from build123d import *

# Parameters (mm, degrees)
SKETCH1_R           = 1.5
BOSS_EXTRUDE1_DEPTH = 27.5
SKETCH1_3_R         = 3.5
BOSS_EXTRUDE2_DEPTH = 18
FILLET1_R           = 0.3
CUT_EXTRUDE1_START  = 6
SKETCH2_W           = 18
SKETCH2_H           = 4.33028374
CUT_EXTRUDE1_DEPTH  = 48


with BuildPart() as part:
    # Sketch1 → Boss-Extrude1 (new body)
    with BuildSketch(Plane(origin=(0, 0, 0), x_dir=(0, 0, -1), z_dir=(1, 0, 0))):
        with BuildLine():
            Line((-0.4375, 4.980822598), (-40.13125, 1.494246779))
            ThreePointArc((-40.13125, 1.494246779), (-38.986805794, 1.10609109), (-38.5, 0))
            ThreePointArc((-38.5, 0), (-38.986805794, -1.10609109), (-40.13125, -1.494246779))
            Line((-40.13125, -1.494246779), (-0.4375, -4.980822598))
            ThreePointArc((-0.4375, -4.980822598), (-5, 0), (-0.4375, 4.980822598))
        make_face()
        with Locations((-40, 0)):
            Circle(SKETCH1_R)
    extrude(amount=BOSS_EXTRUDE1_DEPTH)

    # Sketch1_3 → Boss-Extrude2 (add)
    with BuildSketch(Plane(origin=(0, 0, 0), x_dir=(0, 0, -1), z_dir=(1, 0, 0))):
        with BuildLine():
            Line((-0.4375, 4.980822598), (-40.13125, 1.494246779))
            ThreePointArc((-40.13125, 1.494246779), (-41.5, 0), (-40.13125, -1.494246779))
            Line((-40.13125, -1.494246779), (-0.4375, -4.980822598))
            ThreePointArc((-0.4375, -4.980822598), (5, 0), (-0.4375, 4.980822598))
        make_face()
        Circle(SKETCH1_3_R, mode=Mode.SUBTRACT)
    extrude(amount=-BOSS_EXTRUDE2_DEPTH)

    # Fillet1
    fillet1_edges = [part.edges().sort_by_distance(p)[0] for p in [
        (13.75, 4.980822598, 0.4375),
        (13.75, -4.980822598, 0.4375),
    ]]
    fillet(fillet1_edges, radius=FILLET1_R)

    # Sketch2 → Cut-Extrude1 (cut)
    with BuildSketch(Plane.XY.offset(CUT_EXTRUDE1_START)):
        with Locations((-9, -3.96514187)):
            Rectangle(SKETCH2_W, SKETCH2_H)
    extrude(amount=CUT_EXTRUDE1_DEPTH, mode=Mode.SUBTRACT)


solid = part.part
Design review of the part built by this model. Coordinates are the model's own, in mm. A direction names the side the tool comes from. Round coordinates to 2 decimals unless told otherwise and drop trailing zeros. Write each loop counter-clockwise with the first axis right and the second up, starting at its lowest first coordinate (ties: lowest second). Pieces come first, ordered by that corner, then holes.
Item 1: Consider section A-A on x = -10.5. Give the boundary of the cut face in (y, z).
Item 2: For pin 1 Ø5 at (y, z) = (1.5, 1.5) entering from +X; pin 2 Ø1.5 at (x, z) = (10.5, 13.5) entering from -Y; pin 3 Ø14.5 at (x, z) = (-13, 14.5) entering from -Y; pin 4 Ø4 at (x, z) = (13.5, 0.5) entering from -Y, all flat-tipped, find the tip position at first contact; note any pin that passes through.
Item 3: Consider section D-D on z = 18. Give the boundary of the cut face in (x, y).
Item 4: Consider section C-C on y = -2.75. Give the boundary of the cut face in (x, z).
Item 5: Consider section B-B on y = 0. Give the boundary of the cut face in (x, z), and give its area (3 significant figures).
Item 6: Wall thickness on L1, parallel to Y at x = -12, z = 0; L2, parallel to X at y = -4, z = 0; L3, parallel to Y at x = -10.5, z = -1.5: over which ranges is each line inside the solid? List them lowest first.
Item 7: Draft analysis for pull direction Z (two halves, no side actions). For faces 4 (the cylindrical face through (-8.874, -1.341, -3.233)), 5 (the flat face through (-18, 0, 19)), 6 (the flat face through (-9, -3, 6)), state which applies: released by +Z, released by -Z, zero draft, split by the parting line, or undercut.
Item 8: For faces 1 (the flat face through (0, 3.4, -2.2)), 2 (the flat face through (10.124, -3.213, 20.562)), 3 (the flat face through (0, -3, 14)), list the 3-axis set-ups (+Z, -Z, +X, -X, +Y, -Y) from which the entire face can be reached by the end or side of a thin tool; tool diameter is ignored.
Check values:
1. outline: (-4.98, 0.44) arc R5 ccw (long way) to (4.98, 0.44) - (1.49, 40.13) arc R1.5 ccw to (-1.49, 40.13) - (-1.8, 36.65) - (-1.8, 6) - (-4.49, 6) - close; hole circle Ø7 at (0, 0)
2. pin 1: stops at x = 0
2. pin 2: stops at y = -3.9
2. pin 3: stops at y = -1.8
2. pin 4: passes through
3. outline: (-18, -1.8) - (0, -1.8) - (0, -3.44) - (27.5, -3.44) - (27.5, 3.44) - (-18, 3.44) - close
4. outline: (-18, -4.18) - (0, -4.18) - (0, -2.17) - (-18, -2.17) - close; (-18, 2.17) - (0, 2.17) - (0, 4.18) - (27.5, 4.18) - (27.5, 25.83) - (0, 25.83) - (0, 6) - (-18, 6) - close
5. outline: (-18, -5) - (0, -5) - (0, -3.5) - (-18, -3.5) - close; (-18, 3.5) - (0, 3.5) - (0, 5) - (27.5, 5) - (27.5, 41.5) - (-18, 41.5) - close
5. area: 1,710 mm2
6. L1: y = -5 to -3.5, 3.5 to 5
6. L2: x = -18 to 0
6. L3: y = -4.77 to -3.16, 3.16 to 4.77
7. face 4: undercut
7. face 5: zero draft
7. face 6: released by +Z
8. face 1: -Z, +X
8. face 2: +Z, +X, -X, -Y
8. face 3: +Z, -X, -Y
